from build123d import *

# Parameters (mm, degrees)
SKETCH1_R                    = 50
BOSS_EXTRUDE1_DEPTH          = 5
F_10_2_10_2_DIAMETER_HOLE1_D = 10.2
M3_CLEARANCE_HOLE1_D         = 3.4
CUT_EXTRUDE2_DEPTH           = 5
CUT_EXTRUDE3_DEPTH           = 10
FILLET1_R                    = 1
SKETCH13_R                   = 10
CUT_EXTRUDE4_DEPTH           = 10


with BuildPart() as part:
    # Sketch1 → Boss-Extrude1 (new body)
    with BuildSketch(Plane.XY):
        Circle(SKETCH1_R)
    extrude(amount=BOSS_EXTRUDE1_DEPTH)

    # Ø10.2 (10.2) Diameter Hole1 (through all)
    with Locations(Plane(origin=(0, 0, 0), x_dir=(-1, 0, 0), z_dir=(0, 0, -1))):
        with Locations((37, 0), (-37, 0), (0, -40)):
            Hole(F_10_2_10_2_DIAMETER_HOLE1_D / 2)

    # M3 Clearance Hole1 (through all)
    with Locations(Plane.XY.offset(5)):
        with Locations((46, 0), (28, 0), (9, -40), (-9, -40), (-46, 0), (-28, 0)):
            Hole(M3_CLEARANCE_HOLE1_D / 2)

    # Sketch11 → Cut-Extrude2 (cut)
    with BuildSketch(Plane.XY.offset(5)):
        with BuildLine():
            Line((22, 22.5), (32, 22.5))
            ThreePointArc((32, 22.5), (32.707106781, 22.792893219), (33, 23.5))
            Line((33, 23.5), (33, 26.5))
            ThreePointArc((33, 26.5), (32.707106781, 27.207106781), (32, 27.5))
            Line((32, 27.5), (22, 27.5))
            ThreePointArc((22, 27.5), (21.292893219, 27.207106781), (21, 26.5))
            Line((21, 26.5), (21, 23.5))
            ThreePointArc((21, 23.5), (21.292893219, 22.792893219), (22, 22.5))
        make_face()
        with BuildLine():
            Line((-22, 27.5), (-32, 27.5))
            ThreePointArc((-32, 27.5), (-32.707106781, 27.207106781), (-33, 26.5))
            Line((-33, 26.5), (-33, 23.5))
            ThreePointArc((-33, 23.5), (-32.707106781, 22.792893219), (-32, 22.5))
            Line((-32, 22.5), (-22, 22.5))
            ThreePointArc((-22, 22.5), (-21.292893219, 22.792893219), (-21, 23.5))
            Line((-21, 23.5), (-21, 26.5))
            ThreePointArc((-21, 26.5), (-21.292893219, 27.207106781), (-22, 27.5))
        make_face()
        with BuildLine():
            Line((-21, -27.5), (-21, -30.5))
            ThreePointArc((-21, -30.5), (-21.292893219, -31.207106781), (-22, -31.5))
            Line((-22, -31.5), (-32, -31.5))
            ThreePointArc((-32, -31.5), (-32.707106781, -31.207106781), (-33, -30.5))
            Line((-33, -30.5), (-33, -27.5))
            ThreePointArc((-33, -27.5), (-32.707106781, -26.792893219), (-32, -26.5))
            Line((-32, -26.5), (-22, -26.5))
            ThreePointArc((-22, -26.5), (-21.292893219, -26.792893219), (-21, -27.5))
        make_face()
        with BuildLine():
            Line((22, -31.5), (32, -31.5))
            ThreePointArc((32, -31.5), (32.707106781, -31.207106781), (33, -30.5))
            Line((33, -30.5), (33, -27.5))
            ThreePointArc((33, -27.5), (32.707106781, -26.792893219), (32, -26.5))
            Line((32, -26.5), (22, -26.5))
            ThreePointArc((22, -26.5), (21.292893219, -26.792893219), (21, -27.5))
            Line((21, -27.5), (21, -30.5))
            ThreePointArc((21, -30.5), (21.292893219, -31.207106781), (22, -31.5))
        make_face()
    extrude(amount=-CUT_EXTRUDE2_DEPTH, mode=Mode.SUBTRACT)

    # Sketch12 → Cut-Extrude3 (cut)
    with BuildSketch(Plane.XY.offset(5)):
        with BuildLine():
            Line((-6, 33), (6, 33))
            ThreePointArc((6, 33), (8.121320344, 33.878679656), (9, 36))
            Line((9, 36), (9, 50))
            Line((9, 50), (-9, 50))
            Line((-9, 50), (-9, 36))
            ThreePointArc((-9, 36), (-8.121320344, 33.878679656), (-6, 33))
        make_face()
    extrude(amount=-CUT_EXTRUDE3_DEPTH, mode=Mode.SUBTRACT)

    # Fillet1
    fillet1_edges = [part.edges().sort_by_distance(p)[0] for p in [
        (-9, 49.183330509, 2.5),
        (9, 49.183330509, 2.5),
    ]]
    fillet(fillet1_edges, radius=FILLET1_R)

    # Sketch13 → Cut-Extrude4 (cut)
    with BuildSketch(Plane.XY.offset(5)):
        Circle(SKETCH13_R)
    extrude(amount=-CUT_EXTRUDE4_DEPTH, mode=Mode.SUBTRACT)


solid = part.part
Verification items for the finished model (mm, model axes). A direction names the side the tool comes from. Coordinates: 2 decimals unless noted, no trailing zeros. Loops run counter-clockwise (first coordinate to the right, second up) from the corner with the lowest first, then second, coordinate; pieces in that order, holes last. Notation, with made-up numbers: M -8,31.25 L 18,31.25 A13 cw 18,45.25 Z; hole C 21.25,8.5 d7. An arc over 180 degrees is marked long. One line per item, written item: value.
1. Section check D-D on x = -27.5. Record the cut outline in (y, z).
Answers follow:
outline: M -41.76,0 L -31.5,0 L -31.5,5 L -41.76,5 Z; M -26.5,0 L -1.62,0 L -1.62,5 L -26.5,5 Z; M 1.62,0 L 22.5,0 L 22.5,5 L 1.62,5 Z; M 27.5,0 L 41.76,0 L 41.76,5 L 27.5,5 Z
2. Mould release check, pull along X, two halves, no side actions. Record for faces 3 (the flat face through (-27, 22.5, 3)), 4 (the flat face through (10.4, 0.2, 0)): pulls with the +X half, pulls with the -X half, needs draft (parallel to the pull), parting line crosses it, or undercut.
Answers follow:
face 3: undercut
face 4: needs draft
3. Set-up check for faces 1 (the flat face through (9, 42, 3)), 2 (the flat face through (33, -29, 3)): record each of +Z, -Z, +X, -X, +Y, -Y from which the full face is reachable in a straight line by a thin tool's end or side.
Answers follow:
face 1: +Z, -Z, +Y
face 2: +Z, -Z
4. Section check C-C on y = 0. Give the number of separate pieces and of enclosed holes in the cut face, plus the area to 3 significant figures.
Answers follow:
separate pieces: 8
enclosed holes: 0
area: 230 mm^2
5. Section check B-B on x = 1.5. Record the cut outline in (y, z), plus the area to 3 significant figures.
Answers follow:
outline: M -49.98,0 L -44.87,0 L -44.87,5 L -49.98,5 Z; M -35.13,0 L -9.89,0 L -9.89,5 L -35.13,5 Z; M 9.89,0 L 33,0 L 33,5 L 9.89,5 Z
area: 267 mm^2
6. Material ranges on line 1 along Y through (x, z) = (-4, 3.15); line 2 along Y through (x, z) = (7.5, 0.3); line 3 along X through (y, z) = (-27.5, 1.35), recorded low to high. Write a range as from..to.
Answers follow:
line 1: -49.84..-43.16, -36.84..-9.17, 9.17..33
line 2: -49.43..-40.8, -39.2..-6.61, 6.61..33.4
line 3: -41.76..-33, -21..21, 33..41.76
7. Section check A-A on y = -40. Record the cut outline in (x, z).
Answers follow:
outline: M -30,0 L -10.7,0 L -10.7,5 L -30,5 Z; M -7.3,0 L -5.1,0 L -5.1,5 L -7.3,5 Z; M 5.1,0 L 7.3,0 L 7.3,5 L 5.1,5 Z; M 10.7,0 L 30,0 L 30,5 L 10.7,5 Z
8. Gauge pin test, flat ends, axial feed: P1, Ø2, axis at x = -28, y = 0, coming from the -Z side; P2, Ø1, axis at y = 37, z = 1, coming from the +X side; P3, Ø2.5, axis at y = -29.5, z = 1.5, coming from the +X side; P4, Ø2.5, axis at x = 25.5, z = 3, coming from the -Y side. Record the tip position at first contact, or that the pin passes through.
Answers follow:
P1: through
P2: x = 34.17
P3: x = 41.25
P4: y = -43.73
